Verification items for this drawing (mm, ordinates from the low corner). Coordinates: 2 decimals unless noted, no trailing zeros. Write each loop counter-clockwise with the first axis right and the second up, starting at its lowest first coordinate (ties: lowest second). Pieces come first, ordered by that corner, then holes.
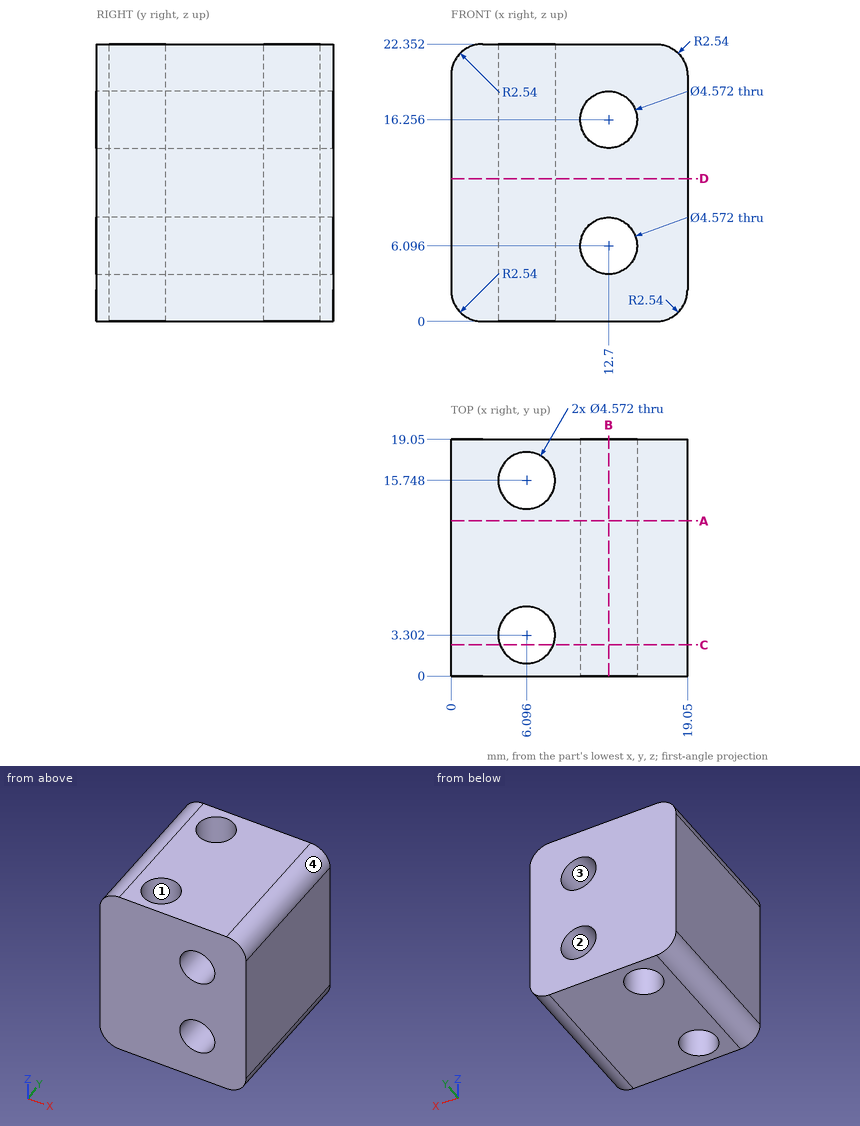
1. Gauge pin test, flat end, axial feed: pin 1 Ø1.5 at (x, z) = (11.5, 18) entering from -Y. Record the tip position at first contact, or that the pin passes through.
Computed values:
pin 1: stops at y = 0
2. Thickness scan on line 1 along Y through (x, z) = (6.25, 11.5); line 2 along Y through (x, z) = (4, 20); line 3 along X through (y, z) = (16.5, 4.5). Record the ranges inside material, lowest first.
Computed values:
line 1: y = 0 to 1.02, 5.58 to 13.47, 18.03 to 19.05
line 2: y = 0 to 2.39, 4.21 to 14.84, 16.66 to 19.05
line 3: x = 0 to 3.94, 8.25 to 11.06, 14.34 to 19.05
3. Sectioned sample at C-C, the plane y = 2.5. Record the boundary of the cut face in (x, z).
Computed values:
outline: (0, 2.54) arc R2.54 ccw to (2.54, 0) - (3.96, 0) - (3.96, 22.35) - (2.54, 22.35) arc R2.54 ccw to (0, 19.81) - close; (8.24, 0) - (16.51, 0) arc R2.54 ccw to (19.05, 2.54) - (19.05, 19.81) arc R2.54 ccw to (16.51, 22.35) - (8.24, 22.35) - close; hole circle Ø4.57 at (12.7, 6.1); hole circle Ø4.57 at (12.7, 16.26)
4. Sectioned sample at A-A, the plane y = 12.5. Record the boundary of the cut face in (x, z), and give its area (3 significant figures).
Computed values:
outline: (0, 2.54) arc R2.54 ccw to (2.54, 0) - (16.51, 0) arc R2.54 ccw to (19.05, 2.54) - (19.05, 19.81) arc R2.54 ccw to (16.51, 22.35) - (2.54, 22.35) arc R2.54 ccw to (0, 19.81) - close; hole circle Ø4.57 at (12.7, 6.1); hole circle Ø4.57 at (12.7, 16.26)
area: 387 mm2
5. Sectioned sample at B-B, the plane x = 12.7. Record the boundary of the cut face in (y, z), and give its area (3 significant figures).
Computed values:
outline: (0, 0) - (19.05, 0) - (19.05, 3.81) - (0, 3.81) - close; (0, 8.38) - (19.05, 8.38) - (19.05, 13.97) - (0, 13.97) - close; (0, 18.54) - (19.05, 18.54) - (19.05, 22.35) - (0, 22.35) - close
area: 252 mm2
6. Sectioned sample at D-D, the plane z = 11.5. Record the boundary of the cut face in (x, y), and give its area (3 significant figures).
Computed values:
outline: (0, 0) - (19.05, 0) - (19.05, 19.05) - (0, 19.05) - close; hole circle Ø4.57 at (6.1, 3.3); hole circle Ø4.57 at (6.1, 15.75)
area: 330 mm2
7. Draft check along Z on the marked faces 1, 2, 3 and 4. Enter one of: released by +Z, released by -Z, zero draft, split by the parting line, or undercut.
Computed values:
face 1: zero draft
face 2: undercut
face 3: undercut
face 4: released by +Z
